Read the model definition and answer for the solid it produces. Units are mm, in the model's axes. Face numbers are marked on the shaded views. A direction names the side the tool comes from. Coordinates: 2 decimals unless noted, no trailing zeros. Order: outer loops, then holes, each group sorted by start corner. A loop starts at its lowest first (then second) coordinate and runs counter-clockwise, first axis right, second up. Notation, with made-up numbers: M -1.5,1.25 L 6.5,1.25 A18 cw 6.5,33.25 Z; hole C -2,3 d2. An arc over 180 degrees is marked long. Use a Markdown table: item, result. Add a question column.
1) The mould has two halves that part along Z. Classify the marked faces 1, 2, 3 and 4: released by +Z, released by -Z, zero draft, split by the parting line, or undercut.
2) This flat-tipped pin is pushed along its axis until it touches: pin 1 Ø15 at (x, z) = (0, -52) entering from +Y. Where does it stop, or does it pass through?
3) For the marked faces 5 and 6, determine the directions among +Z, -Z, +X, -X, +Y, -Y from which every point of the face is accessible in a straight line to the end or side of a thin tool.
4) Find the intervals of material crossed by probe 1 along X at (y, z) = (13.5, 0); probe 2 along X at (y, z) = (21.5, 4.5); probe 3 along Z at (x, y) = (-4, 20), in increasing order. Write a range as [from, to].
5) Find section B-B on y = 10.5. Count the separate pieces of the cut face and the enclosed holes in it, plus the area to 3 significant figures.
6) Find section C-C on z = -52. Write down the section's boundary in (x, y), plus the area to 3 significant figures.
7) Find section A-A on x = 26. Write down the section's boundary in (y, z), plus the area to 3 significant figures.
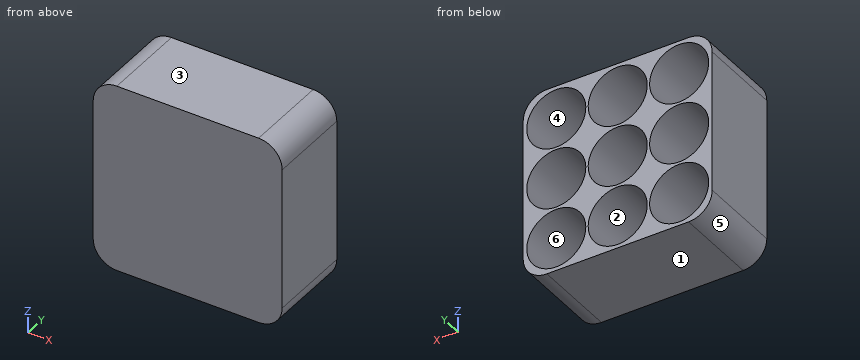
from build123d import *

# Parameters (mm, degrees)
SKETCH2_W           = 80
SKETCH2_H           = 80
SKETCH2_R           = 12.5
BOSS_EXTRUDE2_DEPTH = 35
SKETCH3_W           = 80
SKETCH3_H           = 80
BOSS_EXTRUDE3_DEPTH = 1
FILLET1_R           = 10


with BuildPart() as part:
    # Sketch2 → Boss-Extrude2 (new body)
    with BuildSketch(Plane(origin=(0, 0, 0), x_dir=(1, 0, 0), z_dir=(0, 1, 0))):
        with Locations((26, 26)):
            Rectangle(SKETCH2_W, SKETCH2_H)
        with Locations(Location((0, 0, 0), (0, 0, 270))):
            Circle(SKETCH2_R, mode=Mode.SUBTRACT)
        with Locations(Location((26, 0, 0), (0, 0, 270))):
            Circle(SKETCH2_R, mode=Mode.SUBTRACT)
        with Locations(Location((52, 0, 0), (0, 0, 270))):
            Circle(SKETCH2_R, mode=Mode.SUBTRACT)
        with Locations(Location((26, 26, 0), (0, 0, 270))):
            Circle(SKETCH2_R, mode=Mode.SUBTRACT)
        with Locations(Location((52, 26, 0), (0, 0, 270))):
            Circle(SKETCH2_R, mode=Mode.SUBTRACT)
        with Locations(Location((26, 52, 0), (0, 0, 270))):
            Circle(SKETCH2_R, mode=Mode.SUBTRACT)
        with Locations(Location((52, 52, 0), (0, 0, 270))):
            Circle(SKETCH2_R, mode=Mode.SUBTRACT)
        with Locations(Location((0, 26, 0), (0, 0, 270))):
            Circle(SKETCH2_R, mode=Mode.SUBTRACT)
        with Locations(Location((0, 52, 0), (0, 0, 270))):
            Circle(SKETCH2_R, mode=Mode.SUBTRACT)
    extrude(amount=BOSS_EXTRUDE2_DEPTH)

    # Sketch3 → Boss-Extrude3 (add)
    with BuildSketch(Plane.XZ):
        with Locations((26, -26)):
            Rectangle(SKETCH3_W, SKETCH3_H)
    extrude(amount=BOSS_EXTRUDE3_DEPTH)

    # Fillet1
    fillet1_edges = [part.edges().sort_by_distance(p)[0] for p in [
        (66, 17, 14),
        (-14, 17, 14),
        (-14, 17, -66),
        (66, 17, -66),
    ]]
    fillet(fillet1_edges, radius=FILLET1_R)


solid = part.part
Check result:
| question | item | result |
|---|---|---|
| 1 | face 1 | released by -Z |
| 1 | face 2 | undercut |
| 1 | face 3 | released by +Z |
| 1 | face 4 | undercut |
| 2 | pin 1 | stops at y = 0 |
| 3 | face 5 | -Z, -X, +Y, -Y |
| 3 | face 6 | +Y |
| 4 | probe 1 | x = [-14, -12.5], [12.5, 13.5], [38.5, 39.5], [64.5, 66] |
| 4 | probe 2 | x = [-13.99, -11.66], [11.66, 14.34], [37.66, 40.34], [63.66, 65.99] |
| 4 | probe 3 | z = [-66, -63.84], [-40.16, -37.84], [-14.16, -11.84], [11.84, 14] |
| 5 | separate pieces | 1 |
| 5 | enclosed holes | 9 |
| 5 | area | 1,900 mm2 |
| 6 | outline | M -14,-1 L 66,-1 L 66,35 L 64.5,35 L 64.5,0 L 39.5,0 L 39.5,35 L 38.5,35 L 38.5,0 L 13.5,0 L 13.5,35 L 12.5,35 L 12.5,0 L -12.5,0 L -12.5,35 L -14,35 Z |
| 6 | area | 255 mm2 |
| 7 | outline | M -1,-66 L 35,-66 L 35,-64.5 L 0,-64.5 L 0,-39.5 L 35,-39.5 L 35,-38.5 L 0,-38.5 L 0,-13.5 L 35,-13.5 L 35,-12.5 L 0,-12.5 L 0,12.5 L 35,12.5 L 35,14 L -1,14 Z |
| 7 | area | 255 mm2 |
